Part model, mm, in its own coordinate system. Give positions to 0.01 mm unless a question says otherwise; leave off trailing zeros. Order: outer loops, then holes, each group sorted by start corner. A loop starts at its lowest first (then second) coordinate and runs counter-clockwise, first axis right, second up. Notation, with made-up numbers: M 70.5,47 L 75.5,47 A15 cw 75.5,65 Z; hole C -33.5,29 d6. An arc over 180 degrees is marked long. Return JSON: item names as keys, results as strings.
from build123d import *

# Parameters (mm, degrees)
SKETCH2_R           = 18.5
SKETCH2_W           = 22.5
SKETCH2_H           = 22.5
BOSS_EXTRUDE1_DEPTH = 2.5
SKETCH4_R           = 1.67
CUT_EXTRUDE1_DEPTH  = 1.15
CIRPATTERN1_COUNT   = 4
SKETCH5_W           = 22.5
SKETCH5_H           = 22.5
SKETCH5_W_2         = 19
SKETCH5_H_2         = 19
BOSS_EXTRUDE2_DEPTH = 0.6
FILLET1_R           = 1
SKETCH6_R           = 1.5
CUT_EXTRUDE2_DEPTH  = 1.9


with BuildPart() as part:
    # Sketch2 → Boss-Extrude1 (new body)
    with BuildSketch(Plane(origin=(0, 0, 0), x_dir=(1, 0, 0), z_dir=(0, 1, 0))):
        with Locations(Location((-21.383734207, -0.621346489, 0), (0, 0, 270))):
            Circle(SKETCH2_R)
        with Locations((-21.383734207, -0.621346489)):
            Rectangle(SKETCH2_W, SKETCH2_H, mode=Mode.SUBTRACT)
    extrude(amount=BOSS_EXTRUDE1_DEPTH)

    # Sketch4 → Cut-Extrude1 (cut)
    with BuildSketch(Plane.XZ):
        with Locations(Location((-21.569675845, 16.401346489, 0), (0, 0, 270))):
            Circle(SKETCH4_R)
    cut_extrude1 = extrude(amount=-CUT_EXTRUDE1_DEPTH, mode=Mode.SUBTRACT)

    # CirPattern1: Cut-Extrude1 ×4 about axis
    cirpattern1_axis = Axis((-21.383734207, 0, 0.621346489), (0, 1, 0))
    for i in range(1, CIRPATTERN1_COUNT):
        add(cut_extrude1.rotate(cirpattern1_axis, i * 360 / CIRPATTERN1_COUNT), mode=Mode.SUBTRACT)

    # Sketch5 → Boss-Extrude2 (add)
    with BuildSketch(Plane(origin=(0, 2.5, 0), x_dir=(1, 0, 0), z_dir=(0, 1, 0))):
        with Locations((-21.383734207, -0.621346489)):
            Rectangle(SKETCH5_W, SKETCH5_H)
        with Locations((-21.383734207, -0.621346489)):
            Rectangle(SKETCH5_W_2, SKETCH5_H_2, mode=Mode.SUBTRACT)
    extrude(amount=-BOSS_EXTRUDE2_DEPTH)

    # Fillet1
    fillet1_edges = [part.edges().sort_by_distance(p)[0] for p in [
        (-30.883734207, 2.2, -8.878653511),
        (-30.883734207, 2.2, 10.121346489),
        (-11.883734207, 2.2, 10.121346489),
        (-11.883734207, 2.2, -8.878653511),
    ]]
    fillet(fillet1_edges, radius=FILLET1_R)

    # Sketch6 → Cut-Extrude2 (cut)
    with BuildSketch(Plane(origin=(0, 0, 0), x_dir=(-1, 0, 0), z_dir=(0, -1, 0))):
        with Locations((32.133734207, -11.371346489)):
            Circle(SKETCH6_R)
        with Locations((10.633734207, -11.371346489)):
            Circle(SKETCH6_R)
        with Locations((10.633734207, 10.128653511)):
            Circle(SKETCH6_R)
        with Locations((32.133734207, 10.128653511)):
            Circle(SKETCH6_R)
    extrude(amount=-CUT_EXTRUDE2_DEPTH, mode=Mode.SUBTRACT)


solid = part.part
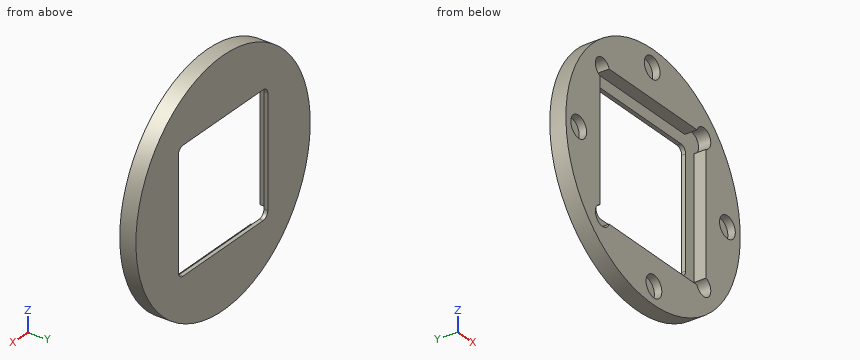
Q1. Pin check, flat tips, straight feed: pin 1 (5 mm diameter, centred on x = -26, z = 6, fed in from +Y); pin 2 (1 mm diameter, centred on y = 1.5, z = 8.5, fed in from +X); pin 3 (1 mm diameter, centred on y = 0.5, z = -2, fed in from +X); pin 4 (1.5 mm diameter, centred on x = -11, y = 2, fed in from -Z). Stop position of each tip, or through.
Established:
{"pin 1": "passes through", "pin 2": "stops at x = -4.42", "pin 3": "stops at x = -3.01", "pin 4": "stops at z = -15.17"}
Q2. Band-saw the part on D-D (z = -15). Give the cut face in (x, y).
Established:
{"outline": "M -31.29,0 L -22.86,0 L -22.86,1.15 L -19.54,1.15 L -19.54,0 L -11.47,0 L -11.47,2.5 L -31.29,2.5 Z"}
Q3. Probe line 1 along Z through (x, y) = (-9.5, 0.7); line 2 along Z through (x, y) = (-27.5, 0.65); line 3 along Z through (x, y) = (-33, 0.5). List the from-to ranges inside material, lowest first.
Established:
{"line 1": "z = -13.56 to -11.11, -9.15 to 10.39, 12.35 to 14.8", "line 2": "z = -16.84 to -10.63, 11.87 to 18.08", "line 3": "z = -13.78 to -11.35, -8.9 to 10.15, 12.6 to 15.02"}
Q4. Band-saw the part on C-C (y = 0.5). Give the cut face in (x, z), then the cut area to 3 significant figures.
Established:
{"outline": "C -21.38,0.62 d37; hole C -37.16,0.44 d3.34; hole M -32.63,-8.71 A1.5 ccw long -30.72,-10.63 L -12.05,-10.63 A1.5 ccw long -10.13,-8.71 L -10.13,9.96 A1.5 ccw long -12.05,11.87 L -30.72,11.87 A1.5 ccw long -32.63,9.96 Z; hole C -21.57,16.4 d3.34; hole C -21.2,-15.16 d3.34; hole C -5.6,0.81 d3.34", "area": "520 mm²"}
Q5. Band-saw the part on A-A (x = -17). Give the cut face in (y, z), then the cut area to 3 significant figures.
Established:
{"outline": "M 0,-17.35 L 2.5,-17.35 L 2.5,-8.88 L 1.9,-8.88 L 1.9,-10.63 L 0,-10.63 Z; M 0,11.87 L 1.9,11.87 L 1.9,10.12 L 2.5,10.12 L 2.5,18.59 L 0,18.59 Z", "area": "35.7 mm²"}
Q6. Band-saw the part on B-B (z = 6). Give the cut face in (x, y), then the cut area to 3 significant figures.
Established:
{"outline": "M -39.08,0 L -32.63,0 L -32.63,1.9 L -30.88,1.9 L -30.88,2.5 L -39.08,2.5 Z; M -11.88,1.9 L -10.13,1.9 L -10.13,0 L -3.68,0 L -3.68,2.5 L -11.88,2.5 Z", "area": "34.4 mm²"}
